Geometry: final body of the model. Coordinates: model frame, mm. Give positions to 0.01 mm unless a question says otherwise; leave off trailing zeros. Write each loop counter-clockwise with the first axis right and the second up, starting at its lowest first coordinate (ties: lowest second). Pieces come first, ordered by that corner, then holes. Notation, with made-up numbers: (-1, 16) - (52, 16) arc R27 ccw to (52, 36) - close; hole circle Ø5 at (9, 88). An arc over 180 degrees is marked (long way). Use CSV: the item, a comma, the result in double quotes. Start each with the question number.
(1) Line query: probe 1 along X at (y, z) = (37, 26.5); probe 2 along X at (y, z) = (40, 31); probe 3 along Z at (x, y) = (17.5, -13). Output: solid intervals per line, ascending. Write a range as [from, to].
(2) Section A-A on z = 26. Output: boundary loops of the cut face in (x, y), and give its area (3 significant figures).
(3) Section C-C on x = 0. Output: boundary loops of the cut face in (y, z) (1 decimal).
(4) Section D-D on z = 10. Output: boundary loops of the cut face in (x, y).
(5) Draft query along X for faces 1 (the cylindrical face through (-0.782, -0.711, 36.504)), 2 (the flat face through (0, 50.8, 38)), 3 (the cylindrical face through (0.884, -0.711, 41.266)). Return one class per face: released by +X, released by -X, zero draft, split by the parting line, or undercut.
(6) First-contact query: pin 1 Ø2 at (y, z) = (-28, 5.5) entering from +X; pin 2 Ø2 at (y, z) = (40.5, 20) entering from -X; pin 3 Ø6 at (x, y) = (21, 22.5) entering from -Z. Flat tips, straight axial feed; report the tip coordinate or a pass-through.
from build123d import *

# Parameters (mm, degrees)
F1_DEPTH = 50.8
F2_R     = 1.5875


with BuildPart() as f1:
    # F0 (on Front) → F1 (new body, symmetric)
    with BuildSketch(Plane.XZ):
        with BuildLine():
            ThreePointArc((-36.5125, 0), (0, 36.5125), (36.5125, 0))
            Line((36.5125, 0), (41.275, 0))
            ThreePointArc((41.275, 0), (0, 41.275), (-41.275, 0))
            Line((-41.275, 0), (-36.5125, 0))
        make_face()
    extrude(amount=F1_DEPTH, both=True)

    # F2
    f2_edges = [f1.edges().sort_by_distance(p)[0] for p in [
        (-41.275, 0, 0),
        (-36.5125, 0, 0),
        (36.5125, 0, 0),
        (41.275, 0, 0),
    ]]
    fillet(f2_edges, radius=F2_R)


solid = f1.part
Check values:
1,probe 1,"x = [-31.64, -25.12], [25.12, 31.64]"
1,probe 2,"x = [-27.25, -19.29], [19.29, 27.25]"
1,probe 3,"z = [32.05, 37.38]"
2,outline,"(-32.06, -50.8) - (-25.64, -50.8) - (-25.64, 50.8) - (-32.06, 50.8) - close; (25.64, -50.8) - (32.06, -50.8) - (32.06, 50.8) - (25.64, 50.8) - close"
2,area,"1,300 mm²"
3,outline,"(-50.8, 36.5) - (50.8, 36.5) - (50.8, 41.3) - (-50.8, 41.3) - close"
4,outline,"(-40.05, -50.8) - (-35.12, -50.8) - (-35.12, 50.8) - (-40.05, 50.8) - close; (35.12, -50.8) - (40.05, -50.8) - (40.05, 50.8) - (35.12, 50.8) - close"
5,face 1,"undercut"
5,face 2,"zero draft"
5,face 3,"split by the parting line"
6,pin 1,"stops at x = 41.03"
6,pin 2,"stops at x = -36.64"
6,pin 3,"stops at z = 27.52"
